```python
from build123d import *

# Parameters (mm, degrees)
F1_DEPTH = 3.42
F2_R     = 2
F4_D     = 8
F5_D     = 8.5
F6_D     = 6.5
F7_D     = 7.14
F8_D     = 5.5


with BuildPart() as f1:
    # F0 (on Front) → F1 (new body)
    with BuildSketch(Plane.XZ):
        Polygon((-80, -10), (-80, -100), (80, -100), (80, -10), (88, -10), (88, 10), (80, 10), (80, 100), (45, 100), (45, 155), (-45, 155), (-45, 100), (-80, 100), (-80, 10), (-88, 10), (-88, -10), align=None)
        with BuildLine():
            ThreePointArc((-26.32, 41.47), (-23.57, 44.22), (-20.82, 41.47))
            Line((-20.82, 41.47), (-20.82, 37.47))
            ThreePointArc((-20.82, 37.47), (-23.57, 34.72), (-26.32, 37.47))
            Line((-26.32, 37.47), (-26.32, 41.47))
        make_face(mode=Mode.SUBTRACT)
        with BuildLine():
            ThreePointArc((-26.32, 88.57), (-23.57, 91.32), (-20.82, 88.57))
            Line((-20.82, 88.57), (-20.82, 84.57))
            ThreePointArc((-20.82, 84.57), (-23.57, 81.82), (-26.32, 84.57))
            Line((-26.32, 84.57), (-26.32, 88.57))
        make_face(mode=Mode.SUBTRACT)
        with BuildLine():
            ThreePointArc((-26.32, 101.47), (-23.57, 104.22), (-20.82, 101.47))
            Line((-20.82, 101.47), (-20.82, 97.47))
            ThreePointArc((-20.82, 97.47), (-23.57, 94.72), (-26.32, 97.47))
            Line((-26.32, 97.47), (-26.32, 101.47))
        make_face(mode=Mode.SUBTRACT)
        with BuildLine():
            ThreePointArc((-26.32, 148.57), (-23.57, 151.32), (-20.82, 148.57))
            Line((-20.82, 148.57), (-20.82, 144.57))
            ThreePointArc((-20.82, 144.57), (-23.57, 141.82), (-26.32, 144.57))
            Line((-26.32, 144.57), (-26.32, 148.57))
        make_face(mode=Mode.SUBTRACT)
        with BuildLine():
            ThreePointArc((20.78, 41.47), (23.53, 44.22), (26.28, 41.47))
            Line((26.28, 41.47), (26.28, 37.47))
            ThreePointArc((26.28, 37.47), (23.53, 34.72), (20.78, 37.47))
            Line((20.78, 37.47), (20.78, 41.47))
        make_face(mode=Mode.SUBTRACT)
        with BuildLine():
            ThreePointArc((20.78, 88.57), (23.53, 91.32), (26.28, 88.57))
            Line((26.28, 88.57), (26.28, 84.57))
            ThreePointArc((26.28, 84.57), (23.53, 81.82), (20.78, 84.57))
            Line((20.78, 84.57), (20.78, 88.57))
        make_face(mode=Mode.SUBTRACT)
        with BuildLine():
            Line((-19.75, 120.82), (-19.75, 124.82))
            ThreePointArc((-19.75, 124.82), (0, 144.57), (19.75, 124.82))
            Line((19.75, 124.82), (19.75, 120.82))
            ThreePointArc((19.75, 120.82), (0, 101.07), (-19.75, 120.82))
        make_face(mode=Mode.SUBTRACT)
        with BuildLine():
            ThreePointArc((20.78, 101.47), (23.53, 104.22), (26.28, 101.47))
            Line((26.28, 101.47), (26.28, 97.47))
            ThreePointArc((26.28, 97.47), (23.53, 94.72), (20.78, 97.47))
            Line((20.78, 97.47), (20.78, 101.47))
        make_face(mode=Mode.SUBTRACT)
        with BuildLine():
            ThreePointArc((20.78, 148.57), (23.53, 151.32), (26.28, 148.57))
            Line((26.28, 148.57), (26.28, 144.57))
            ThreePointArc((26.28, 144.57), (23.53, 141.82), (20.78, 144.57))
            Line((20.78, 144.57), (20.78, 148.57))
        make_face(mode=Mode.SUBTRACT)
    extrude(amount=F1_DEPTH)

    # F2
    f2_edges = [f1.edges().sort_by_distance(p)[0] for p in [
        (45, -1.71, 155),
        (45, -1.71, 100),
        (80, -1.71, 100),
        (-45, -1.71, 100),
        (-80, -1.71, 100),
        (-80, -1.71, 10),
        (-88, -1.71, 10),
        (-88, -1.71, -10),
        (-80, -1.71, -10),
        (-80, -1.71, -100),
        (80, -1.71, -100),
        (80, -1.71, -10),
        (88, -1.71, -10),
        (88, -1.71, 10),
        (80, -1.71, 10),
    ]]
    fillet(f2_edges, radius=F2_R)

    # F4 (through all)
    with Locations(Plane.XZ.offset(3.42)):
        with Locations((-28, 27), (28, 27), (28, -48), (-28, -48)):
            Hole(F4_D / 2)

    # F5 (through all)
    with Locations(Plane.XZ.offset(3.42)):
        with Locations((-13, 19.5), (13, 19.5)):
            Hole(F5_D / 2)

    # F6 (through all)
    with Locations(Plane.XZ.offset(3.42)):
        with Locations((-53.5, 89), (53.5, 89), (-53.5, -91), (53.5, -91), (0, -87)):
            Hole(F6_D / 2)

    # F7 (through all)
    with Locations(Plane.XZ.offset(3.42)):
        with Locations((-72, -87), (72, -87)):
            Hole(F7_D / 2)

    # F8 (through all)
    with Locations(Plane.XZ.offset(3.42)):
        with Locations((-37, 148.65), (37, 148.65), (37, 106.35), (-37, 106.35), (-72, 92.5), (-72, 66.25), (-72, 20), (-72, 46.25), (72, 46.25), (72, 20), (72, 66.25), (72, 92.5)):
            Hole(F8_D / 2)


solid = f1.part
```
Geometry check sheet. Reference: the model listing, model coordinates, mm. Give positions to 0.01 mm unless a question says otherwise; leave off trailing zeros. Write each loop counter-clockwise with the first axis right and the second up, starting at its lowest first coordinate (ties: lowest second). Pieces come first, ordered by that corner, then holes. Notation, with made-up numbers: (74, 6.5) -> (95, 6.5) arc R31 cw to (95, 45.5) -> close; hole circle Ø4 at (59, -17). An arc over 180 degrees is marked (long way). Use one line per item in the form item = value.
Item 1: Depth check by flat-ended pin: pin 1 Ø1 at (x, y) = (-57, -0.5) entering from +Z; pin 2 Ø1.7 at (y, z) = (-1.5, 99) entering from +X. Enter the tip coordinate at first touch or a pass-through.
Results list:
pin_1 = 100
pin_2 = 79.99
Item 2: Scan lines: line 1 (Z direction, x = -28, y = -0.65); line 2 (Z direction, x = 72, y = -2.25); line 3 (Z direction, x = 22, y = -1.3). Record each from-to range of solid material in increasing order.
Results list:
line_1 = -100 to -52, -44 to 23, 31 to 155
line_2 = -100 to -90.57, -83.43 to 17.25, 22.75 to 43.5, 49 to 63.5, 69 to 89.75, 95.25 to 100
line_3 = -100 to 35.18, 43.76 to 82.28, 90.86 to 95.18, 103.76 to 142.28, 150.86 to 155
Item 3: Sectioned sample at D-D on x = -11.5. Enter the section's corners in (y, z), plus the area to 3 significant figures.
Results list:
outline = (-3.42, -100) -> (0, -100) -> (0, 15.52) -> (-3.42, 15.52) -> close; (-3.42, 23.48) -> (0, 23.48) -> (0, 104.76) -> (-3.42, 104.76) -> close; (-3.42, 140.88) -> (0, 140.88) -> (0, 155) -> (-3.42, 155) -> close
area = 721 mm2
Item 4: Sectioned sample at B-B on x = -72. Enter the section's corners in (y, z).
Results list:
outline = (-3.42, -100) -> (0, -100) -> (0, -90.57) -> (-3.42, -90.57) -> close; (-3.42, -83.43) -> (0, -83.43) -> (0, 17.25) -> (-3.42, 17.25) -> close; (-3.42, 22.75) -> (0, 22.75) -> (0, 43.5) -> (-3.42, 43.5) -> close; (-3.42, 49) -> (0, 49) -> (0, 63.5) -> (-3.42, 63.5) -> close; (-3.42, 69) -> (0, 69) -> (0, 89.75) -> (-3.42, 89.75) -> close; (-3.42, 95.25) -> (0, 95.25) -> (0, 100) -> (-3.42, 100) -> close
Item 5: Mould release check, pull along X, two halves, no side actions. Record for faces 1 (the flat face through (-1, -3.42, 29)), 2 (the cylindrical face through (-69.973, -1.686, 68.109)): released by +X, released by -X, zero draft, split by the parting line, or undercut.
Results list:
face_1 = zero draft
face_2 = undercut
Item 6: Sectioned sample at A-A on x = -37. Enter the section's corners in (y, z).
Results list:
outline = (-3.42, -100) -> (0, -100) -> (0, 103.6) -> (-3.42, 103.6) -> close; (-3.42, 109.1) -> (0, 109.1) -> (0, 145.9) -> (-3.42, 145.9) -> close; (-3.42, 151.4) -> (0, 151.4) -> (0, 155) -> (-3.42, 155) -> close
Item 7: Sectioned sample at C-C on y = -2.4. Count the separate pieces of the cut face and the enclosed holes in it, plus the area to 3 significant figures.
Results list:
separate_pieces = 1
enclosed_holes = 34
area = 34,700 mm2
